from build123d import *

# Parameters (mm, degrees)
F2_R     = 4.6355
F3_DEPTH = 13.97
F4_R     = 1.5875
F5_DEPTH = 20.32


with BuildPart() as f1:
    # F0 (on Front) → F1 (revolve)
    with BuildSketch(Plane.XZ):
        Polygon((0, 58.42), (0, 0), (30.48, 26.67), (30.48, 39.37), (12.7, 39.37), (12.7, 58.42), align=None)
    revolve(axis=Axis((0, 0, 29.21), (0, 0, -1)))

    # F2 (on face) → F3 (cut)
    with BuildSketch(Plane.XY.offset(58.42)):
        Circle(F2_R)
    extrude(amount=-F3_DEPTH, mode=Mode.SUBTRACT)

    # F4 (on Top) → F5 (cut)
    with BuildSketch(Plane.XY):
        Circle(F4_R)
    extrude(amount=F5_DEPTH, mode=Mode.SUBTRACT)


solid = f1.part
The model under review builds one solid part; all positions refer to its coordinate system, in mm. A direction names the side the tool comes from. Give positions to 0.01 mm unless a question says otherwise; leave off trailing zeros. Order: outer loops, then holes, each group sorted by start corner. A loop starts at its lowest first (then second) coordinate and runs counter-clockwise, first axis right, second up. Notation, with made-up numbers: M 43,15.5 L 59,15.5 A25 cw 59,42.5 Z; hole C -5.5,-30.5 d3. An arc over 180 degrees is marked long. Use one line per item in the form item = value. Start each with the question number.
Item 1: We need section A-A on x = 0. Give the boundary of the cut face in (y, z).
Item 2: We need section C-C on z = 43. Give the boundary of the cut face in (x, y), plus the area to 3 significant figures.
Item 3: To check wall thickness, follow line 1 along Y through (x, z) = (0, 51.25); line 2 along X through (y, z) = (0, 14); line 3 along X through (y, z) = (3, 47.5). State the ranges of each line that lie inside material, in increasing order. Write a range as from..to.
Item 4: For faces 1 (the flat face through (0, 0, 44.45)), 2 (the flat face through (0, 0, 20.32)), list the 3-axis set-ups (+Z, -Z, +X, -X, +Y, -Y) from which the entire face can be reached by the end or side of a thin tool; tool diameter is ignored.
Item 5: Insertion check: pin 1 Ø3 at (x, z) = (6.5, 18.5) entering from -Y; pin 2 Ø4.5 at (x, y) = (-1, 2) entering from +Z; pin 3 Ø12 at (y, z) = (4, 46.5) entering from -X; pin 4 Ø3.5 at (x, y) = (0.5, -0.5) entering from -Z. Each pin has a flat end and moves straight along its axis. Give the tip position at first contact, or say it passes through.
Item 6: The part is to be moulded in two halves that separate along X. For faces 3 (the cylindrical face through (-6.607, 29.755, 33.109)), 4 (the flat face through (5, 0, 58.42)), 5 (the cylindrical face through (-3.42, 3.13, 51.53)), say which applies: pulls with the +X half, pulls with the -X half, needs draft (parallel to the pull), parting line crosses it, or undercut.
Item 7: We need section D-D on z = 33. Give the boundary of the cut face in (x, y).
Completed:
q1.outline = M -30.48,26.67 L -1.59,1.39 L -1.59,20.32 L 1.59,20.32 L 1.59,1.39 L 30.48,26.67 L 30.48,39.37 L 12.7,39.37 L 12.7,58.42 L 4.64,58.42 L 4.64,44.45 L -4.64,44.45 L -4.64,58.42 L -12.7,58.42 L -12.7,39.37 L -30.48,39.37 Z
q2.outline = C 0,0 d25.4
q2.area = 507 mm²
q3.line_1 = -12.7..-4.64, 4.64..12.7
q3.line_2 = -16..-1.59, 1.59..16
q3.line_3 = -12.34..-3.53, 3.53..12.34
q4.face_1 = +Z
q4.face_2 = -Z
q5.pin_1 = -21.97
q5.pin_2 = 44.45
q5.pin_3 = -12.7
q5.pin_4 = 1.39
q6.face_3 = parting line crosses it
q6.face_4 = needs draft
q6.face_5 = undercut
q7.outline = C 0,0 d60.96
